from build123d import *

# Parameters (mm, degrees)
BOSS_EXTRUDE1_DEPTH = 2.25
BOSS_EXTRUDE2_DEPTH = 2.5


with BuildPart() as part:
    # Sketch1 → Boss-Extrude1 (new body)
    with BuildSketch(Plane.XY.offset(30)):
        with BuildLine():
            Line((-291, 3.75), (-291, -100.25))
            ThreePointArc((-291, -100.25), (-289.389087297, -104.139087297), (-285.5, -105.75))
            Line((-285.5, -105.75), (30.5, -105.75))
            Line((30.5, -105.75), (35.5, -105.75))
            Line((35.5, -105.75), (351.5, -105.75))
            ThreePointArc((351.5, -105.75), (355.389087297, -104.139087297), (357, -100.25))
            Line((357, -100.25), (357, 3.75))
            ThreePointArc((357, 3.75), (355.389087297, 7.639087297), (351.5, 9.25))
            Line((351.5, 9.25), (35.5, 9.25))
            Line((35.5, 9.25), (30.5, 9.25))
            Line((30.5, 9.25), (-285.5, 9.25))
            ThreePointArc((-285.5, 9.25), (-289.389087297, 7.639087297), (-291, 3.75))
        make_face()
        with BuildLine():
            Line((30.5, 6.25), (-285.5, 6.25))
            ThreePointArc((-285.5, 6.25), (-287.267766953, 5.517766953), (-288, 3.75))
            Line((-288, 3.75), (-288, -100.25))
            ThreePointArc((-288, -100.25), (-287.267766953, -102.017766953), (-285.5, -102.75))
            Line((-285.5, -102.75), (30.5, -102.75))
            ThreePointArc((30.5, -102.75), (32.267766953, -102.017766953), (33, -100.25))
            ThreePointArc((33, -100.25), (33.732233047, -102.017766953), (35.5, -102.75))
            Line((35.5, -102.75), (351.5, -102.75))
            ThreePointArc((351.5, -102.75), (353.267766953, -102.017766953), (354, -100.25))
            Line((354, -100.25), (354, 3.75))
            ThreePointArc((354, 3.75), (353.267766953, 5.517766953), (351.5, 6.25))
            Line((351.5, 6.25), (35.5, 6.25))
            ThreePointArc((35.5, 6.25), (33.732233047, 5.517766953), (33, 3.75))
            ThreePointArc((33, 3.75), (32.267766953, 5.517766953), (30.5, 6.25))
        make_face(mode=Mode.SUBTRACT)
    extrude(amount=-BOSS_EXTRUDE1_DEPTH)

    # Sketch2 → Boss-Extrude2 (add)
    # profile 1 of 2: a face of its own
    with BuildSketch(Plane(origin=(0, 0, 27.75), x_dir=(-1, 0, 0), z_dir=(0, 0, -1))):
        with BuildLine():
            Line((291, -100.25), (291, 3.75))
            ThreePointArc((291, 3.75), (289.389087297, 7.639087297), (285.5, 9.25))
            Line((285.5, 9.25), (-351.5, 9.25))
            ThreePointArc((-351.5, 9.25), (-355.389087297, 7.639087297), (-357, 3.75))
            Line((-357, 3.75), (-357, -100.25))
            ThreePointArc((-357, -100.25), (-355.389087297, -104.139087297), (-351.5, -105.75))
            Line((-351.5, -105.75), (285.5, -105.75))
            ThreePointArc((285.5, -105.75), (289.389087297, -104.139087297), (291, -100.25))
        make_face()
        with BuildLine():
            ThreePointArc((288, -100.25), (287.267766953, -102.017766953), (285.5, -102.75))
            Line((285.5, -102.75), (-30.5, -102.75))
            ThreePointArc((-30.5, -102.75), (-32.267766953, -102.017766953), (-33, -100.25))
            ThreePointArc((-33, -100.25), (-33.732233047, -102.017766953), (-35.5, -102.75))
            Line((-35.5, -102.75), (-351.5, -102.75))
            ThreePointArc((-351.5, -102.75), (-353.267766953, -102.017766953), (-354, -100.25))
            Line((-354, -100.25), (-354, 3.75))
            ThreePointArc((-354, 3.75), (-353.267766953, 5.517766953), (-351.5, 6.25))
            Line((-351.5, 6.25), (-35.5, 6.25))
            ThreePointArc((-35.5, 6.25), (-33.732233047, 5.517766953), (-33, 3.75))
            ThreePointArc((-33, 3.75), (-32.267766953, 5.517766953), (-30.5, 6.25))
            Line((-30.5, 6.25), (285.5, 6.25))
            ThreePointArc((285.5, 6.25), (287.267766953, 5.517766953), (288, 3.75))
            Line((288, 3.75), (288, -100.25))
        make_face(mode=Mode.SUBTRACT)
    # profile 2 of 2: a face of its own
    with BuildSketch(Plane(origin=(0, 0, 27.75), x_dir=(-1, 0, 0), z_dir=(0, 0, -1))):
        with BuildLine():
            Line((-351, 3.75), (-36, 3.75))
            Line((-36, 3.75), (-36, -100.25))
            Line((-36, -100.25), (-158.5, -100.25))
            Line((-158.5, -100.25), (-158.5, -102.75))
            Line((-158.5, -102.75), (-35.5, -102.75))
            ThreePointArc((-35.5, -102.75), (-33.732233047, -102.017766953), (-33, -100.25))
            ThreePointArc((-33, -100.25), (-32.267766953, -102.017766953), (-30.5, -102.75))
            Line((-30.5, -102.75), (92.5, -102.75))
            Line((92.5, -102.75), (92.5, -100.25))
            Line((92.5, -100.25), (-30, -100.25))
            Line((-30, -100.25), (-30, 3.75))
            Line((-30, 3.75), (285, 3.75))
            Line((285, 3.75), (285, -100.25))
            Line((285, -100.25), (162.5, -100.25))
            Line((162.5, -100.25), (162.5, -102.75))
            Line((162.5, -102.75), (285.5, -102.75))
            ThreePointArc((285.5, -102.75), (287.267766953, -102.017766953), (288, -100.25))
            Line((288, -100.25), (288, 3.75))
            ThreePointArc((288, 3.75), (287.267766953, 5.517766953), (285.5, 6.25))
            Line((285.5, 6.25), (-30.5, 6.25))
            ThreePointArc((-30.5, 6.25), (-32.267766953, 5.517766953), (-33, 3.75))
            ThreePointArc((-33, 3.75), (-33.732233047, 5.517766953), (-35.5, 6.25))
            Line((-35.5, 6.25), (-351.5, 6.25))
            ThreePointArc((-351.5, 6.25), (-353.267766953, 5.517766953), (-354, 3.75))
            Line((-354, 3.75), (-354, -100.25))
            ThreePointArc((-354, -100.25), (-353.267766953, -102.017766953), (-351.5, -102.75))
            Line((-351.5, -102.75), (-228.5, -102.75))
            Line((-228.5, -102.75), (-228.5, -100.25))
            Line((-228.5, -100.25), (-351, -100.25))
            Line((-351, -100.25), (-351, 3.75))
        make_face()
    extrude(amount=BOSS_EXTRUDE2_DEPTH)


solid = part.part
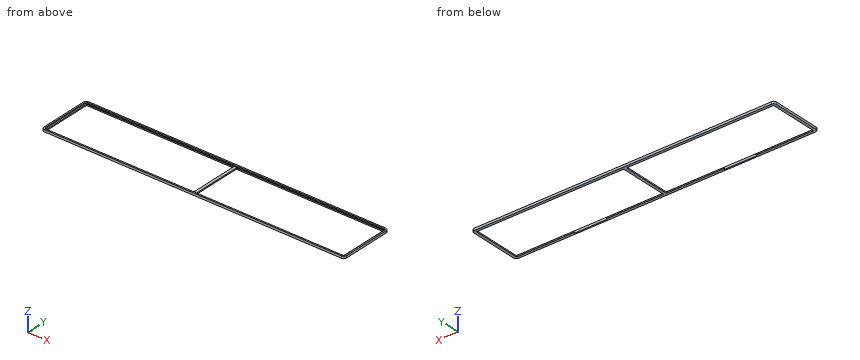
Input: part model. Units: mm. Frame: model coordinates. Give positions to 0.01 mm unless a question says otherwise; leave off trailing zeros. Order: outer loops, then holes, each group sorted by start corner. A loop starts at its lowest first (then second) coordinate and runs counter-clockwise, first axis right, second up. Notation, with made-up numbers: (16.25, 77.5) -> (51.25, 77.5) arc R17 ccw to (51.25, 109.5) -> close; hole circle Ø1 at (-2, 0.5). An arc over 180 degrees is marked (long way). Use one line per item in the form item = value.
1) Section B-B, the plane z = 28.75. Return loops of the section in (x, y).
Response values:
outline = (-291, -100.25) arc R5.5 ccw to (-285.5, -105.75) -> (351.5, -105.75) arc R5.5 ccw to (357, -100.25) -> (357, 3.75) arc R5.5 ccw to (351.5, 9.25) -> (-285.5, 9.25) arc R5.5 ccw to (-291, 3.75) -> close; hole (-288, -100.25) arc R2.5 ccw to (-285.5, -102.75) -> (30.5, -102.75) arc R2.5 ccw to (33, -100.25) arc R2.5 ccw to (35.5, -102.75) -> (351.5, -102.75) arc R2.5 ccw to (354, -100.25) -> (354, 3.75) arc R2.5 ccw to (351.5, 6.25) -> (35.5, 6.25) arc R2.5 ccw to (33, 3.75) arc R2.5 ccw to (30.5, 6.25) -> (-285.5, 6.25) arc R2.5 ccw to (-288, 3.75) -> close
2) Line query: probe 1 along X at (y, z) = (-78.5, 27); probe 2 along X at (y, z) = (-24, 29.2); probe 3 along X at (y, z) = (5.5, 28.95). Output: solid intervals per line, ascending.
Response values:
probe_1 = -291 to -285, 30 to 36, 351 to 357
probe_2 = -291 to -288, 354 to 357
probe_3 = -290.71 to -287.29, 32.29 to 33.71, 353.29 to 356.71
3) Section A-A, the plane x = 206. Return loops of the section in (y, z), and give its area (4 significant figures).
Response values:
outline = (-105.75, 25.25) -> (-102.75, 25.25) -> (-102.75, 30) -> (-105.75, 30) -> close; (3.75, 25.25) -> (9.25, 25.25) -> (9.25, 30) -> (6.25, 30) -> (6.25, 27.75) -> (3.75, 27.75) -> close
area = 34.75 mm^2
4) Section D-D, the plane x = -190. Return loops of the section in (y, z), and give its area (3 significant figures).
Response values:
outline = (-105.75, 25.25) -> (-100.25, 25.25) -> (-100.25, 27.75) -> (-102.75, 27.75) -> (-102.75, 30) -> (-105.75, 30) -> close; (3.75, 25.25) -> (9.25, 25.25) -> (9.25, 30) -> (6.25, 30) -> (6.25, 27.75) -> (3.75, 27.75) -> close
area = 41.0 mm^2
5) Section C-C, the plane y = -17.5. Return loops of the section in (x, z).
Response values:
outline = (-291, 25.25) -> (-285, 25.25) -> (-285, 27.75) -> (-288, 27.75) -> (-288, 30) -> (-291, 30) -> close; (30, 25.25) -> (36, 25.25) -> (36, 27.75) -> (30, 27.75) -> close; (351, 25.25) -> (357, 25.25) -> (357, 30) -> (354, 30) -> (354, 27.75) -> (351, 27.75) -> close
6) First-contact query: pin 1 Ø1.2 at (y, z) = (-101.5, 27) entering from +X; pin 2 Ø0.8 at (y, z) = (-101.5, 26.5) entering from +X; pin 3 Ø1.2 at (y, z) = (-101.5, 26.5) entering from -X. Flat tips, straight axial feed; report the tip coordinate or a pass-through.
Response values:
pin_1 = 356.96
pin_2 = 356.93
pin_3 = -290.96
